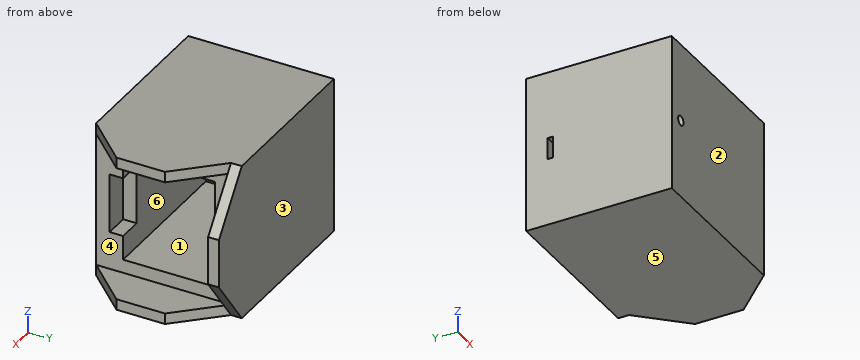
```python
from build123d import *

# Parameters (mm, degrees)
SKETCH_1_W               = 29
SKETCH_1_H               = 29
SKETCH_1_W_2             = 25
SKETCH_1_H_2             = 25
EXTRUDE_1_DEPTH          = 36.2
SKETCH_1_3_W             = 25
SKETCH_1_3_H             = 25
SKETCH_1_3_W_2           = 20
SKETCH_1_3_H_2           = 17
EXTRUDE_2_DEPTH          = 28.6
SKETCH_1_4_W             = 29
SKETCH_1_4_H             = 29
EXTRUDE_3_DEPTH          = 2
SKETCH_1_5_W             = 20
SKETCH_1_5_H             = 17
SKETCH_1_5_W_2           = 8
SKETCH_1_5_H_2           = 8
EXTRUDE_4_DEPTH          = 1.1
CUT_EXTRUDE_1_DEPTH      = 49.597222143
CUT_EXTRUDE_2_REACH      = 49.431
CUT_EXTRUDE_3_DEPTH      = 2
CUT_EXTRUDE_3_DEPTH_BACK = 2
CUT_EXTRUDE_3_START      = -14.5
SKETCH_7_W               = 50
SKETCH_7_H               = 1
HOLE_WIZARD_1_D          = 1.8
HOLE_WIZARD_1_DEPTH      = 4
CUT_EXTRUDE_4_DEPTH      = 4.5


with BuildPart() as part:
    # 草图1 → 凸台-拉伸1 (new body)
    with BuildSketch(Plane(origin=(0, 0, 0), x_dir=(0, 0, -1), z_dir=(1, 0, 0))):
        Rectangle(SKETCH_1_W, SKETCH_1_H)
        Rectangle(SKETCH_1_W_2, SKETCH_1_H_2, mode=Mode.SUBTRACT)
    extrude(amount=EXTRUDE_1_DEPTH)

    # 草图1<3> → 凸台-拉伸2 (add)
    with BuildSketch(Plane(origin=(0, 0, 0), x_dir=(0, 0, -1), z_dir=(1, 0, 0))):
        Rectangle(SKETCH_1_3_W, SKETCH_1_3_H)
        with Locations((0, 1)):
            Rectangle(SKETCH_1_3_W_2, SKETCH_1_3_H_2, mode=Mode.SUBTRACT)
    extrude(amount=EXTRUDE_2_DEPTH)

    # 草图1<4> → 凸台-拉伸3 (add)
    with BuildSketch(Plane(origin=(0, 0, 0), x_dir=(0, 0, -1), z_dir=(1, 0, 0))):
        Rectangle(SKETCH_1_4_W, SKETCH_1_4_H)
    extrude(amount=-EXTRUDE_3_DEPTH)

    # 草图1<5> → 凸台-拉伸4 (add)
    with BuildSketch(Plane(origin=(0, 0, 0), x_dir=(0, 0, -1), z_dir=(1, 0, 0))):
        with Locations((0, 1)):
            Rectangle(SKETCH_1_5_W, SKETCH_1_5_H)
        Rectangle(SKETCH_1_5_W_2, SKETCH_1_5_H_2, mode=Mode.SUBTRACT)
    extrude(amount=EXTRUDE_4_DEPTH)

    # 草图4 → 切除-拉伸1 (cut, through all)
    with BuildSketch(Plane.XY.offset(14.5)):
        Polygon((-2, -12.5), (28.6, -12.5), (36.2, -4.5), (36.2, -14.5), (-2, -14.5), align=None)
        Polygon((36.2, 12.5), (28.6, 12.5), (36.2, 4.5), align=None)
    extrude(amount=-CUT_EXTRUDE_1_DEPTH, mode=Mode.SUBTRACT)

    # 草图6 → 切除-拉伸2 (cut, up to next)
    with BuildSketch(Plane(origin=(0, 14.5, 0), x_dir=(1, 0, 0), z_dir=(0, 1, 0)), mode=Mode.PRIVATE) as cut_extrude_2_sk1:
        Polygon((28.6, 14.5), (36.2, 14.5), (36.2, 4.5), align=None)
    cut_extrude_2_tool1 = extrude(cut_extrude_2_sk1.sketch, amount=-CUT_EXTRUDE_2_REACH, mode=Mode.PRIVATE) & part.part
    # 草图6 → 切除-拉伸2 (cut, up to next)
    with BuildSketch(Plane(origin=(0, 14.5, 0), x_dir=(1, 0, 0), z_dir=(0, 1, 0)), mode=Mode.PRIVATE) as cut_extrude_2_sk2:
        Polygon((36.2, -14.5), (36.2, -4.5), (28.6, -14.5), align=None)
    cut_extrude_2_tool2 = extrude(cut_extrude_2_sk2.sketch, amount=-CUT_EXTRUDE_2_REACH, mode=Mode.PRIVATE) & part.part
    add(cut_extrude_2_tool1.solids().sort_by_distance((33.666667, 14.5, -11.166667))[0], mode=Mode.SUBTRACT)
    add(cut_extrude_2_tool2.solids().sort_by_distance((33.666667, 14.5, 11.166667))[0], mode=Mode.SUBTRACT)

    # 草图7 → 切除-拉伸3 (cut, two sides: drawn at the far end of the back side and taken through both)
    with BuildSketch(Plane.XY.offset(14.5).offset(CUT_EXTRUDE_3_START - CUT_EXTRUDE_3_DEPTH_BACK)):
        with Locations((23, 10)):
            Rectangle(SKETCH_7_W, SKETCH_7_H)
    extrude(amount=CUT_EXTRUDE_3_DEPTH + CUT_EXTRUDE_3_DEPTH_BACK, mode=Mode.SUBTRACT)

    # 孔1
    with Locations(Plane(origin=(0, -12.5, 0), x_dir=(-1, 0, 0), z_dir=(0, -1, 0))):
        with Locations((-1, 0)):
            Hole(HOLE_WIZARD_1_D / 2, depth=HOLE_WIZARD_1_DEPTH)

    # 草图11 → 切除-拉伸4 (cut)
    with BuildSketch(Plane(origin=(28.6, 0, 0), x_dir=(0, 0, -1), z_dir=(1, 0, 0))):
        Polygon((0, -7.5), (-5.5, -7.5), (-5.5, -10), (5.5, -10), (5.5, -7.5), align=None)
    extrude(amount=-CUT_EXTRUDE_4_DEPTH, mode=Mode.SUBTRACT)


solid = part.part
```
CAD build for the part. Positions are in the model's coordinates, mm. Face numbers are marked on the shaded views. A direction names the side the tool comes from. Coordinates: 2 decimals unless noted, no trailing zeros. Order: outer loops, then holes, each group sorted by start corner. A loop starts at its lowest first (then second) coordinate and runs counter-clockwise, first axis right, second up. Notation, with made-up numbers: (56.25, 45) -> (101.25, 45) arc R24 cw to (101.25, 82) -> close; hole circle Ø2 at (48.5, 81.25). An arc over 180 degrees is marked (long way). Use one line per item in the form item = value. Start each with the question number.
1) Pull direction Y, two halves, no side cores. Call the marked faces 1, 2 and 3: +Y half, -Y half, draft (parallel to the pull), parting line (faces both ways), or undercut.
2) Band-saw the part on C-C on z = 7. Give the cut face in (x, y).
3) Drop a flat-ended pin along its axis: pin 1 (12 mm diameter, centred on y = 4, z = 0, fed in from +X). Give the stop position or say it passes through.
4) Drill centre lines: L1, parallel to Z at x = 10.5, y = 0.25; L2, parallel to Z at x = 1, y = -9.3; L3, parallel to Y at x = 23, z = -7.75. Where is each one in solid material? Low to high. Write a range as [from, to].
5) Tool access for the marked faces 4, 5 and 6: list every direction of +Z, -Z, +X, -X, +Y, -Y with a clear straight run to the whole face (end or side of a thin tool).
6) Band-saw the part on B-B on x = 10.5. Give the cut face in (y, z), then the cut area to 3 significant figures.
7) Band-saw the part on D-D on y = 6.5. Give the cut face in (x, z), then the cut area to 3 significant figures.
8) Band-saw the part on A-A on z = 0. Give the cut face in (x, y), then the cut area to 3 significant figures.
Entries:
q1.face_1 = undercut
q1.face_2 = -Y half
q1.face_3 = +Y half
q2.outline = (-2, -12.5) -> (28.6, -12.5) -> (28.6, -7.5) -> (1.1, -7.5) -> (1.1, 9.5) -> (28.6, 9.5) -> (28.6, 12.5) -> (34.3, 12.5) -> (34.3, 14.5) -> (-2, 14.5) -> close
q3.pin_1 = 28.6
q4.L1 = [-14.5, -10], [10, 14.5]
q4.L2 = [-14.5, -0.9], [0.9, 14.5]
q4.L3 = [-12.5, -7.5], [9.5, 14.5]
q5.face_4 = +X, -Y
q5.face_5 = -Z, +X, -X, +Y, -Y
q5.face_6 = +X
q6.outline = (-12.5, -14.5) -> (14.5, -14.5) -> (14.5, 14.5) -> (-12.5, 14.5) -> close; hole (-7.5, -10) -> (9.5, -10) -> (9.5, -2) -> (10.5, -2) -> (10.5, 2) -> (9.5, 2) -> (9.5, 10) -> (-7.5, 10) -> close
q6.area = 439 mm2
q7.outline = (-2, -14.5) -> (34.3, -14.5) -> (34.3, -12.5) -> (28.6, -12.5) -> (28.6, -10) -> (1.1, -10) -> (1.1, 10) -> (28.6, 10) -> (28.6, 12.5) -> (34.3, 12.5) -> (34.3, 14.5) -> (-2, 14.5) -> close
q7.area = 360 mm2
q8.outline = (-2, -12.5) -> (0.1, -12.5) -> (0.1, -8.5) -> (1.9, -8.5) -> (1.9, -12.5) -> (28.6, -12.5) -> (28.6, -10) -> (24.1, -10) -> (24.1, -7.5) -> (1.1, -7.5) -> (1.1, -4) -> (0, -4) -> (0, 4) -> (1.1, 4) -> (1.1, 9.5) -> (-2, 9.5) -> close; (-2, 10.5) -> (28.6, 10.5) -> (28.6, 12.5) -> (36.2, 12.5) -> (36.2, 14.5) -> (-2, 14.5) -> close
q8.area = 316 mm2
